Source: CAD feature listing. Evaluate the final solid. Frame: model axes, mm. Round coordinates to 2 decimals unless told otherwise and drop trailing zeros. Loops run counter-clockwise (first coordinate to the right, second up) from the corner with the lowest first, then second, coordinate; pieces in that order, holes last. Notation, with made-up numbers: M -31,63 L -3,63 A22 ccw -3,69 Z; hole C -17.75,26.25 d2. An arc over 180 degrees is marked long. Answer as a JSON object with one key per item and string values.
from build123d import *

# Parameters (mm, degrees)
SKETCH1_R              = 52
BOSS_EXTRUDE1_DEPTH    = 5
CUT_EXTRUDE1_DEPTH     = 10
SKETCH3_R              = 7.5
CUT_EXTRUDE2_DEPTH     = 10
M3_TAPPED_HOLE3_REACH  = 118.383
M3_TAPPED_HOLE3_BORE_R = 1.25


with BuildPart() as part:
    # Sketch1 → Boss-Extrude1 (new body)
    with BuildSketch(Plane.XY):
        Circle(SKETCH1_R)
    extrude(amount=BOSS_EXTRUDE1_DEPTH)

    # Sketch2 → Cut-Extrude1 (cut)
    with BuildSketch(Plane.XY.offset(5)):
        with BuildLine():
            Line((32, 0), (32, -45))
            Line((32, -45), (42, -45))
            Line((42, -45), (42, 3.54e-07))
            ThreePointArc((42, 3.54e-07), (36.999999823, 5), (32, 0))
        make_face()
        with BuildLine():
            Line((-5, -39.999999646), (-5, -55))
            Line((-5, -55), (5, -55))
            Line((5, -55), (5, -40))
            ThreePointArc((5, -40), (1.77e-07, -35), (-5, -39.999999646))
        make_face()
        with BuildLine():
            Line((-32, -45), (-42, -45))
            Line((-42, -45), (-42, 3.54e-07))
            ThreePointArc((-42, 3.54e-07), (-36.999999823, 5), (-32, 0))
            Line((-32, 0), (-32, -45))
        make_face()
    extrude(amount=-CUT_EXTRUDE1_DEPTH, mode=Mode.SUBTRACT)

    # Sketch3 → Cut-Extrude2 (cut)
    with BuildSketch(Plane.XY.offset(5)):
        Circle(SKETCH3_R)
    extrude(amount=-CUT_EXTRUDE2_DEPTH, mode=Mode.SUBTRACT)

    # M3 Tapped Hole3 bore → M3 Tapped Hole3 (cut, up to next)
    with BuildSketch(Plane(origin=(52, 0, 0), x_dir=(0, 0, -1), z_dir=(1, 0, 0)), mode=Mode.PRIVATE) as m3_tapped_hole3_sk1:
        with Locations((-2.5, 1.82e-07)):
            Circle(M3_TAPPED_HOLE3_BORE_R)
    m3_tapped_hole3_tool1 = extrude(m3_tapped_hole3_sk1.sketch, amount=-M3_TAPPED_HOLE3_REACH, mode=Mode.PRIVATE) & part.part
    m3_tapped_hole3 = m3_tapped_hole3_tool1.solids().sort_by_distance((52, 0, 2.5))[0]
    add(m3_tapped_hole3, mode=Mode.SUBTRACT)

    # Mirror1: M3 Tapped Hole3 across plane
    add(m3_tapped_hole3.mirror(Plane(origin=(0, 0, 0), x_dir=(0, 0, 1), z_dir=(1, 0, 0))), mode=Mode.SUBTRACT)


solid = part.part
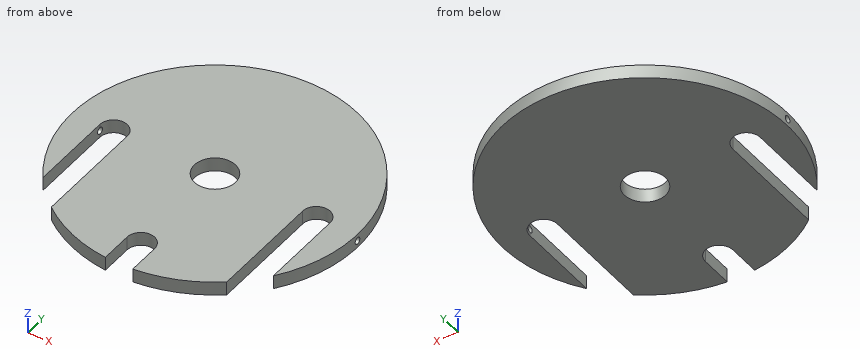
Item 1: Line query: probe 1 along X at (y, z) = (-17, 1.1); probe 2 along X at (y, z) = (2, 3.35); probe 3 along X at (y, z) = (-24, 2.1). Output: solid intervals per line, ascending. Write a range as from..to.
Answer sheet:
{"probe 1": "x = -49.14..-42, -32..32, 42..49.14", "probe 2": "x = -51.96..-41.58, -32.42..-7.23, 7.23..32.42, 41.58..51.96", "probe 3": "x = -46.13..-42, -32..32, 42..46.13"}
Item 2: Section B-B on z = 2.5. Return the cut outline in (x, y).
Answer sheet:
{"outline": "M -51.98,-1.25 A52 ccw -42,-30.66 L -42,-1.25 Z; M -51.98,1.25 L -41.84,1.25 A5 cw -32,0 L -32,-40.99 A52 ccw -5,-51.76 L -5,-40 A5 cw 5,-40 L 5,-51.76 A52 ccw 32,-40.99 L 32,0 A5 cw 41.84,1.25 L 51.98,1.25 A52 ccw Z; M 42,-30.66 A52 ccw 51.98,-1.25 L 42,-1.25 Z; hole C 0,0 d15"}
Item 3: Contact query for flat-ended pins moving along their axis: pin 1 Ø1 at (y, z) = (-19, 3.5) entering from +X; pin 2 Ø3 at (y, z) = (-29.5, 1) entering from +X; pin 3 Ø1 at (y, z) = (-38.5, 4) entering from +X. Output: stop coordinate, or through.
Answer sheet:
{"pin 1": "stops at x = 48.6", "pin 2": "stops at x = 43.82", "pin 3": "stops at x = 32"}
Item 4: Section D-D on y = -24. Return the cut outline in (x, z).
Answer sheet:
{"outline": "M -46.13,0 L -42,0 L -42,5 L -46.13,5 Z; M -32,0 L 32,0 L 32,5 L -32,5 Z; M 42,0 L 46.13,0 L 46.13,5 L 42,5 Z"}
Item 5: Section A-A on x = 0. Return the cut outline in (y, z).
Answer sheet:
{"outline": "M -35,0 L -7.5,0 L -7.5,5 L -35,5 Z; M 7.5,0 L 52,0 L 52,5 L 7.5,5 Z"}
Item 6: Section C-C on y = -3.5. Return the cut outline in (x, z), then the cut area to 3 significant figures.
Answer sheet:
{"outline": "M -51.88,0 L -42,0 L -42,5 L -51.88,5 Z; M -32,0 L -6.63,0 L -6.63,5 L -32,5 Z; M 6.63,0 L 32,0 L 32,5 L 6.63,5 Z; M 42,0 L 51.88,0 L 51.88,5 L 42,5 Z", "area": "352 mm²"}
